Geometry: see drawing. Coordinates: mm, zero at the bounding-box minimum. Give positions to 0.01 mm unless a question says otherwise; leave off trailing zeros. Write each loop counter-clockwise with the first axis right and the second up, starting at its lowest first coordinate (ties: lowest second). Pieces come first, ordered by that corner, then holes. Notation, with made-up numbers: (15.25, 76) - (27.25, 76) arc R18 cw to (27.25, 83) - close; hole circle Ø11 at (-35, 86.25). An arc over 180 degrees is marked (long way). Use a Markdown table: item, result. Add a question column.
1. Section query A-A, the plane x = 6.5. Return loops of the section in (y, z), plus the area to 3 significant figures.
2. Section query D-D, the plane y = 11. Return loops of the section in (x, z).
3. Mould query, pull axis X, two halves, no side actions, for the marked faces 1, 2, 3 and 4. Classes: released by +X, released by -X, zero draft, split by the parting line, or undercut.
4. Section query C-C, the plane z = 78. Return loops of the section in (x, y), plus the area to 3 significant figures.
5. Pin query (flat end, axial travel): pin 1 (2 mm diameter, centred on x = 29.5, z = 65, fed in from +Y). Return the tip coordinate at first contact, or that it passes through.
6. Section query B-B, the plane y = 36.5. Return loops of the section in (x, z), plus the area to 3 significant figures.
7. Material intervals for probe 1 along Z at (x, y) = (6.5, 14); probe 2 along Z at (x, y) = (4, 33); probe 3 along X at (y, z) = (30.5, 57), sorted ascending.
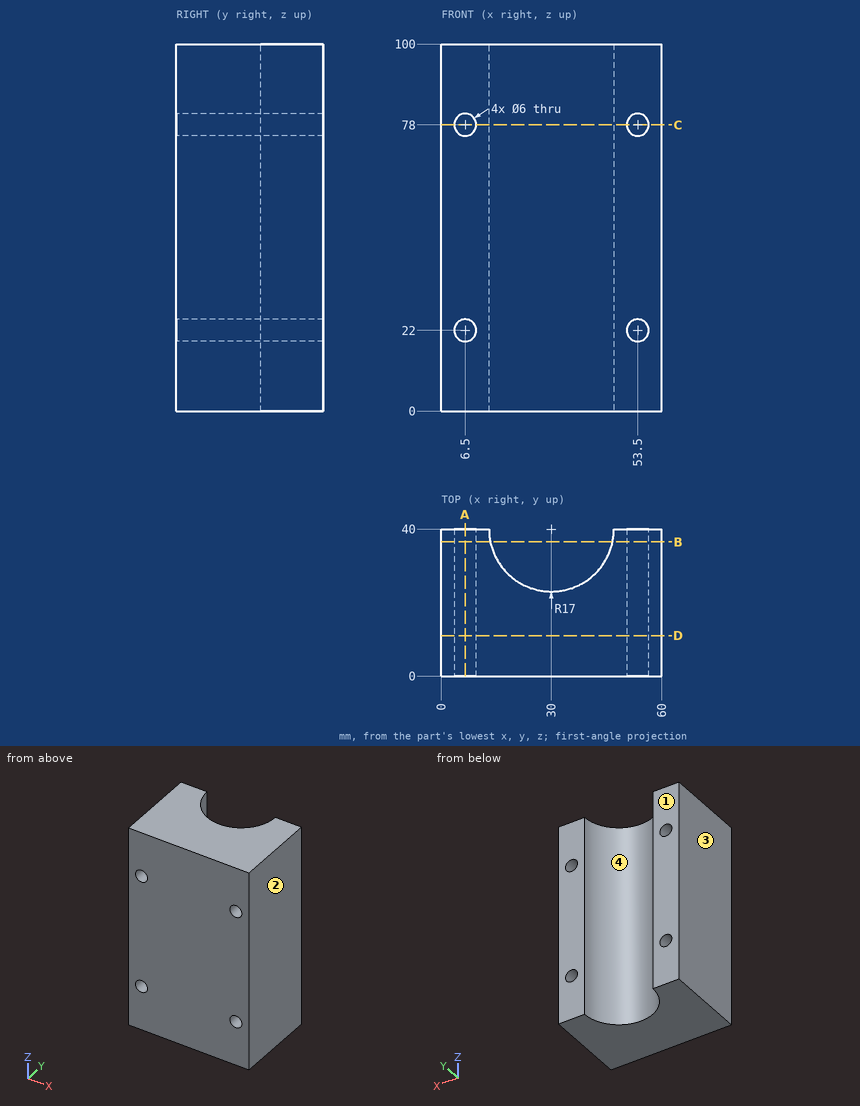
Result sheet:
| question | item | result |
|---|---|---|
| 1 | outline | (0, 0) - (40, 0) - (40, 19) - (0, 19) - close; (0, 25) - (40, 25) - (40, 75) - (0, 75) - close; (0, 81) - (40, 81) - (40, 100) - (0, 100) - close |
| 1 | area | 3,520 mm² |
| 2 | outline | (0, 0) - (60, 0) - (60, 100) - (0, 100) - close; hole circle Ø6 at (6.5, 22); hole circle Ø6 at (6.5, 78); hole circle Ø6 at (53.5, 22); hole circle Ø6 at (53.5, 78) |
| 3 | face 1 | zero draft |
| 3 | face 2 | released by +X |
| 3 | face 3 | released by -X |
| 3 | face 4 | undercut |
| 4 | outline | (0, 0) - (3.5, 0) - (3.5, 40) - (0, 40) - close; (9.5, 0) - (50.5, 0) - (50.5, 40) - (47, 40) arc R17 cw to (13, 40) - (9.5, 40) - close; (56.5, 0) - (60, 0) - (60, 40) - (56.5, 40) - close |
| 4 | area | 1,470 mm² |
| 5 | pin 1 | stops at y = 23.07 |
| 6 | outline | (0, 0) - (13.36, 0) - (13.36, 100) - (0, 100) - close; (46.64, 0) - (60, 0) - (60, 100) - (46.64, 100) - close; hole circle Ø6 at (6.5, 22); hole circle Ø6 at (6.5, 78); hole circle Ø6 at (53.5, 22); hole circle Ø6 at (53.5, 78) |
| 6 | area | 2,560 mm² |
| 7 | probe 1 | z = 0 to 19, 25 to 75, 81 to 100 |
| 7 | probe 2 | z = 0 to 20.34, 23.66 to 76.34, 79.66 to 100 |
| 7 | probe 3 | x = 0 to 15.9, 44.1 to 60 |
